from build123d import *

# Parameters (mm, degrees)
SKETCH1_W            = 137
SKETCH1_H            = 86
SKETCH1_W_2          = 131
SKETCH1_H_2          = 80
BOSS_EXTRUDE1_DEPTH  = 164
SKETCH2_W            = 125
SKETCH2_H            = 152
CUT_EXTRUDE1_DEPTH   = 3
BOSS_EXTRUDE2_DEPTH  = 3
BOSS_EXTRUDE3_DEPTH  = 3
SKETCH3_W            = 152
SKETCH3_H            = 74
CUT_EXTRUDE2_DEPTH   = 3
BOSS_EXTRUDE4_DEPTH  = 3
BOSS_EXTRUDE5_DEPTH  = 3
SKETCH4_W            = 152
SKETCH4_H            = 74
CUT_EXTRUDE3_DEPTH   = 3
BOSS_EXTRUDE6_DEPTH  = 3
BOSS_EXTRUDE7_DEPTH  = 3
SKETCH6_W            = 62.23
SKETCH6_H            = 86
BOSS_EXTRUDE8_DEPTH  = 3
SKETCH7_W            = 62.77
SKETCH7_H            = 152
CUT_EXTRUDE4_DEPTH   = 3
BOSS_EXTRUDE9_DEPTH  = 3
BOSS_EXTRUDE10_DEPTH = 3
SKETCH8_R            = 12.5
SKETCH8_R_2          = 10
BOSS_EXTRUDE11_DEPTH = 32
SKETCH8_4_R          = 10
CUT_EXTRUDE8_DEPTH   = 32
SKETCH9_W            = 6
SKETCH9_H            = 15
BOSS_EXTRUDE12_DEPTH = 15
SKETCH9_3_W          = 6
SKETCH9_3_H          = 15
BOSS_EXTRUDE13_DEPTH = 12
SKETCH9_4_W          = 6
SKETCH9_4_H          = 15
BOSS_EXTRUDE14_DEPTH = 15
FILLET1_R            = 3
SKETCH9_5_W          = 6
SKETCH9_5_H          = 28.664942424
BOSS_EXTRUDE17_DEPTH = 3
SKETCH16_R           = 2
CUT_EXTRUDE13_DEPTH  = 64
SKETCH11_W           = 15
SKETCH11_H           = 10
BOSS_EXTRUDE18_DEPTH = 45
SKETCH18_R           = 1
CUT_EXTRUDE14_DEPTH  = 10
SKETCH19_W           = 15
SKETCH19_H           = 45
BOSS_EXTRUDE19_DEPTH = 2
SKETCH20_R           = 1.65
CUT_EXTRUDE15_DEPTH  = 2
SKETCH21_W           = 15
SKETCH21_H           = 45
BOSS_EXTRUDE20_DEPTH = 9
SKETCH21_3_R         = 3.25
CUT_EXTRUDE16_DEPTH  = 9
SKETCH25_W           = 15
SKETCH25_H           = 45
SKETCH25_R           = 5.5
BOSS_EXTRUDE21_DEPTH = 7.5


with BuildPart() as part:
    # Sketch1 → Boss-Extrude1 (new body)
    with BuildSketch(Plane.XY):
        with Locations((68.5, -43)):
            Rectangle(SKETCH1_W, SKETCH1_H)
        with Locations((68.5, -43)):
            Rectangle(SKETCH1_W_2, SKETCH1_H_2, mode=Mode.SUBTRACT)
    extrude(amount=BOSS_EXTRUDE1_DEPTH)

    # Sketch2 → Cut-Extrude1 (cut)
    with BuildSketch(Plane.XZ.offset(86)):
        with Locations((68.5, 82)):
            Rectangle(SKETCH2_W, SKETCH2_H)
    extrude(amount=-CUT_EXTRUDE1_DEPTH, mode=Mode.SUBTRACT)

    # Sketch2<3> → Boss-Extrude2 (add)
    with BuildSketch(Plane.XZ.offset(86)):
        Polygon((0, 158), (131, 0), (137, 6), (6, 164), align=None)
    extrude(amount=-BOSS_EXTRUDE2_DEPTH)

    # Sketch2<4> → Boss-Extrude3 (add)
    with BuildSketch(Plane.XZ.offset(86)):
        Polygon((131, 164), (0, 6), (6, 0), (137, 158), align=None)
    extrude(amount=-BOSS_EXTRUDE3_DEPTH)

    # Sketch3 → Cut-Extrude2 (cut)
    with BuildSketch(Plane(origin=(137, 0, 0), x_dir=(0, 0, -1), z_dir=(1, 0, 0))):
        with Locations((-82, -43)):
            Rectangle(SKETCH3_W, SKETCH3_H)
    extrude(amount=-CUT_EXTRUDE2_DEPTH, mode=Mode.SUBTRACT)

    # Sketch3<3> → Boss-Extrude4 (add)
    with BuildSketch(Plane(origin=(137, 0, 0), x_dir=(0, 0, -1), z_dir=(1, 0, 0))):
        Polygon((-164, -6), (-6, -86), (0, -80), (-158, 0), align=None)
    extrude(amount=-BOSS_EXTRUDE4_DEPTH)

    # Sketch3<5> → Boss-Extrude5 (add)
    with BuildSketch(Plane(origin=(137, 0, 0), x_dir=(0, 0, -1), z_dir=(1, 0, 0))):
        Polygon((-158, -86), (0, -6), (-6, 0), (-164, -80), align=None)
    extrude(amount=-BOSS_EXTRUDE5_DEPTH)

    # Sketch4 → Cut-Extrude3 (cut)
    with BuildSketch(Plane.ZY):
        with Locations((82, -43)):
            Rectangle(SKETCH4_W, SKETCH4_H)
    extrude(amount=-CUT_EXTRUDE3_DEPTH, mode=Mode.SUBTRACT)

    # Sketch4<4> → Boss-Extrude6 (add)
    with BuildSketch(Plane.ZY):
        Polygon((158, 0), (0, -80), (6, -86), (164, -6), align=None)
    extrude(amount=-BOSS_EXTRUDE6_DEPTH)

    # Sketch4<5> → Boss-Extrude7 (add)
    with BuildSketch(Plane.ZY):
        Polygon((6, 0), (164, -80), (158, -86), (0, -6), align=None)
    extrude(amount=-BOSS_EXTRUDE7_DEPTH)

    # Sketch6 → Boss-Extrude8 (add)
    with BuildSketch(Plane(origin=(0, 0, 0), x_dir=(-1, 0, 0), z_dir=(0, 0, -1))):
        with Locations((-31.115, -43)):
            Rectangle(SKETCH6_W, SKETCH6_H)
    extrude(amount=-BOSS_EXTRUDE8_DEPTH)

    # Sketch7 → Cut-Extrude4 (cut)
    with BuildSketch(Plane(origin=(0, 0, 0), x_dir=(1, 0, 0), z_dir=(0, 1, 0))):
        with Locations((99.615, -82)):
            Rectangle(SKETCH7_W, SKETCH7_H)
    extrude(amount=-CUT_EXTRUDE4_DEPTH, mode=Mode.SUBTRACT)

    # Sketch7<3> → Boss-Extrude9 (add)
    with BuildSketch(Plane(origin=(0, 0, 0), x_dir=(1, 0, 0), z_dir=(0, 1, 0))):
        Polygon((68.23, 0), (137, -158), (131, -164), (62.23, -6), align=None)
    extrude(amount=-BOSS_EXTRUDE9_DEPTH)

    # Sketch7<4> → Boss-Extrude10 (add)
    with BuildSketch(Plane(origin=(0, 0, 0), x_dir=(1, 0, 0), z_dir=(0, 1, 0))):
        Polygon((131, 0), (62.23, -158), (68.23, -164), (137, -6), align=None)
    extrude(amount=-BOSS_EXTRUDE10_DEPTH)

    # Sketch8 → Boss-Extrude11 (add)
    with BuildSketch(Plane(origin=(0, 0, 0), x_dir=(-1, 0, 0), z_dir=(0, 0, -1))):
        with Locations((-48.64, -48.9)):
            Circle(SKETCH8_R)
        with Locations((-48.64, -48.9)):
            Circle(SKETCH8_R_2, mode=Mode.SUBTRACT)
    extrude(amount=-BOSS_EXTRUDE11_DEPTH)

    # Sketch8<4> → Cut-Extrude8 (cut)
    with BuildSketch(Plane(origin=(0, 0, 0), x_dir=(-1, 0, 0), z_dir=(0, 0, -1))):
        with Locations((-48.64, -48.9)):
            Circle(SKETCH8_4_R)
    extrude(amount=-CUT_EXTRUDE8_DEPTH, mode=Mode.SUBTRACT)

    # Sketch9 → Boss-Extrude12 (add)
    with BuildSketch(Plane.ZY):
        with Locations((55, -48.9)):
            Rectangle(SKETCH9_W, SKETCH9_H)
    extrude(amount=BOSS_EXTRUDE12_DEPTH)

    # Sketch9<3> → Boss-Extrude13 (add)
    with BuildSketch(Plane.ZY):
        with Locations((55, -48.9)):
            Rectangle(SKETCH9_3_W, SKETCH9_3_H)
    extrude(amount=BOSS_EXTRUDE13_DEPTH)

    # Sketch9<4> → Boss-Extrude14 (add)
    with BuildSketch(Plane.ZY):
        with Locations((3, -48.9)):
            Rectangle(SKETCH9_4_W, SKETCH9_4_H)
    extrude(amount=BOSS_EXTRUDE14_DEPTH)

    # Fillet1
    fillet1_edges = [part.edges().sort_by_distance(p)[0] for p in [
        (-15, -56.4, 55),
        (-15, -41.4, 55),
        (-15, -56.4, 3),
        (-15, -41.4, 3),
    ]]
    fillet(fillet1_edges, radius=FILLET1_R)

    # Sketch9<5> → Boss-Extrude17 (add)
    with BuildSketch(Plane.ZY):
        with Locations((55, -42.711986128)):
            Rectangle(SKETCH9_5_W, SKETCH9_5_H)
    extrude(amount=-BOSS_EXTRUDE17_DEPTH)

    # Sketch16 → Cut-Extrude13 (cut)
    with BuildSketch(Plane.XY.offset(58)):
        with Locations((-7.5, -48.9)):
            Circle(SKETCH16_R)
    extrude(amount=-CUT_EXTRUDE13_DEPTH, mode=Mode.SUBTRACT)

    # Sketch11 → Boss-Extrude18 (add)
    with BuildSketch(Plane(origin=(0, 0, 0), x_dir=(1, 0, 0), z_dir=(0, 1, 0))):
        with Locations((7.5, -5)):
            Rectangle(SKETCH11_W, SKETCH11_H)
    extrude(amount=BOSS_EXTRUDE18_DEPTH)

    # Sketch18 → Cut-Extrude14 (cut)
    with BuildSketch(Plane.XY.offset(10)):
        with Locations((7.5, 37)):
            Circle(SKETCH18_R)
    extrude(amount=-CUT_EXTRUDE14_DEPTH, mode=Mode.SUBTRACT)

    # Sketch19 → Boss-Extrude19 (add)
    with BuildSketch(Plane.XY.offset(10)):
        with Locations((7.5, 22.5)):
            Rectangle(SKETCH19_W, SKETCH19_H)
    extrude(amount=BOSS_EXTRUDE19_DEPTH)

    # Sketch20 → Cut-Extrude15 (cut)
    with BuildSketch(Plane.XY.offset(12)):
        with Locations((7.5, 37)):
            Circle(SKETCH20_R)
    extrude(amount=-CUT_EXTRUDE15_DEPTH, mode=Mode.SUBTRACT)

    # Sketch21 → Boss-Extrude20 (add)
    with BuildSketch(Plane.XY.offset(12)):
        with Locations((7.5, 22.5)):
            Rectangle(SKETCH21_W, SKETCH21_H)
    extrude(amount=BOSS_EXTRUDE20_DEPTH)

    # Sketch21<3> → Cut-Extrude16 (cut)
    with BuildSketch(Plane.XY.offset(12)):
        with Locations((7.5, 37)):
            Circle(SKETCH21_3_R)
    extrude(amount=CUT_EXTRUDE16_DEPTH, mode=Mode.SUBTRACT)

    # Sketch25 → Boss-Extrude21 (add)
    with BuildSketch(Plane.XY.offset(21)):
        with Locations((7.5, 22.5)):
            Rectangle(SKETCH25_W, SKETCH25_H)
        with Locations((7.5, 37)):
            Circle(SKETCH25_R, mode=Mode.SUBTRACT)
    extrude(amount=BOSS_EXTRUDE21_DEPTH)


solid = part.part
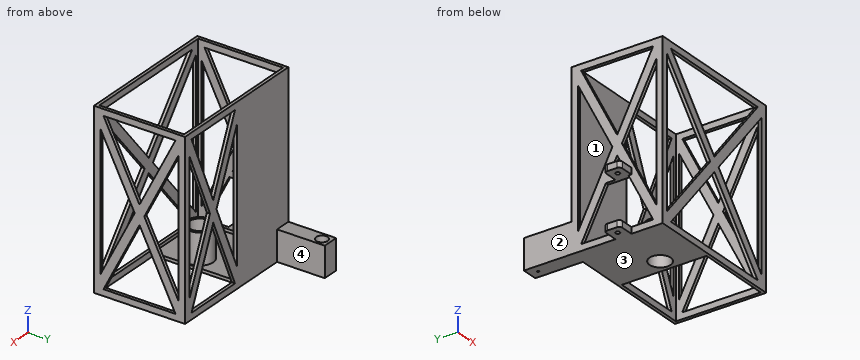
Design review of the part built by this model. Coordinates are the model's own, in mm. Face numbers are marked on the shaded views. Coordinates: 2 decimals unless noted, no trailing zeros. Loops run counter-clockwise (first coordinate to the right, second up) from the corner with the lowest first, then second, coordinate; pieces in that order, holes last. Notation, with made-up numbers: (-33, -6) -> (-1, -6) arc R12 ccw to (-1, 17) -> close; hole circle Ø11 at (77.5, -36.75). An arc over 180 degrees is marked (long way). Use a Markdown table: item, result. Add a question column.
Item 1: Wall thickness on L1, parallel to Y at x = 7, z = 26; L2, parallel to Y at x = -7.5, z = 56.5; L3, parallel to Y at x = 26, z = 100: over which ranges is each line inside the solid? List them lowest first. Write a range as from..to.
Item 2: We need section D-D, the plane y = 7.5. Write out the cut boundary in (x, z), and give its area (4 significant figures).
Item 3: We need section A-A, the plane x = 45. Write out the cut boundary in (y, z), and give its area (3 significant figures).
Item 4: We need section B-B, the plane x = 106. Count the separate pieces of the cut face and the enclosed holes in it, and give its area (3 significant figures).
Item 5: Clearance check with flat-ended pins moving along their axes: P1, Ø5, axis at x = 21, z = 69.5, coming from the -Y side; P2, Ø8, axis at y = -50, z = 23, coming from the -X side; P3, Ø2.5, axis at x = 1.5, z = 87, coming from the +Y side. State where each tip first meets the part, or that it passes through.
Item 6: The part is to be moulded in two halves that separate along X. For the marked faces 1, 2, 3 and 4, say which applies: +X half, -X half, draft (parallel to the pull), parting line (faces both ways), or undercut.
Numbers:
| question | item | result |
|---|---|---|
| 1 | L1 | y = -3..31.52, 42.48..45 |
| 1 | L2 | y = -56.4..-50.9, -46.9..-41.4 |
| 1 | L3 | y = -3..0 |
| 2 | outline | (0, 0) -> (15, 0) -> (15, 28.5) -> (0, 28.5) -> close |
| 2 | area | 427.5 mm^2 |
| 3 | outline | (-86, 0) -> (-58.21, 0) -> (-58.21, 32) -> (-60.86, 32) -> (-60.86, 3) -> (-83, 3) -> (-83, 6) -> (-86, 6) -> close; (-86, 47.04) -> (-83, 47.04) -> (-83, 60.27) -> (-86, 60.27) -> close; (-86, 103.73) -> (-83, 103.73) -> (-83, 116.96) -> (-86, 116.96) -> close; (-86, 158) -> (-83, 158) -> (-83, 164) -> (-86, 164) -> close; (-39.59, 0) -> (0, 0) -> (0, 164) -> (-3, 164) -> (-3, 3) -> (-36.94, 3) -> (-36.94, 32) -> (-39.59, 32) -> close |
| 3 | area | 945 mm^2 |
| 4 | separate pieces | 8 |
| 4 | enclosed holes | 0 |
| 4 | area | 270 mm^2 |
| 5 | P1 | stops at y = -3 |
| 5 | P2 | stops at x = 36.14 |
| 5 | P3 | stops at y = 0 |
| 6 | face 1 | undercut |
| 6 | face 2 | -X half |
| 6 | face 3 | draft |
| 6 | face 4 | +X half |
